Geometry: see drawing. Coordinates: mm, zero at the bounding-box minimum. A direction names the side the tool comes from. Give positions to 0.01 mm unless a question says otherwise; leave off trailing zeros. Write each loop counter-clockwise with the first axis right and the second up, starting at its lowest first coordinate (ties: lowest second). Pieces come first, ordered by that corner, then holes.
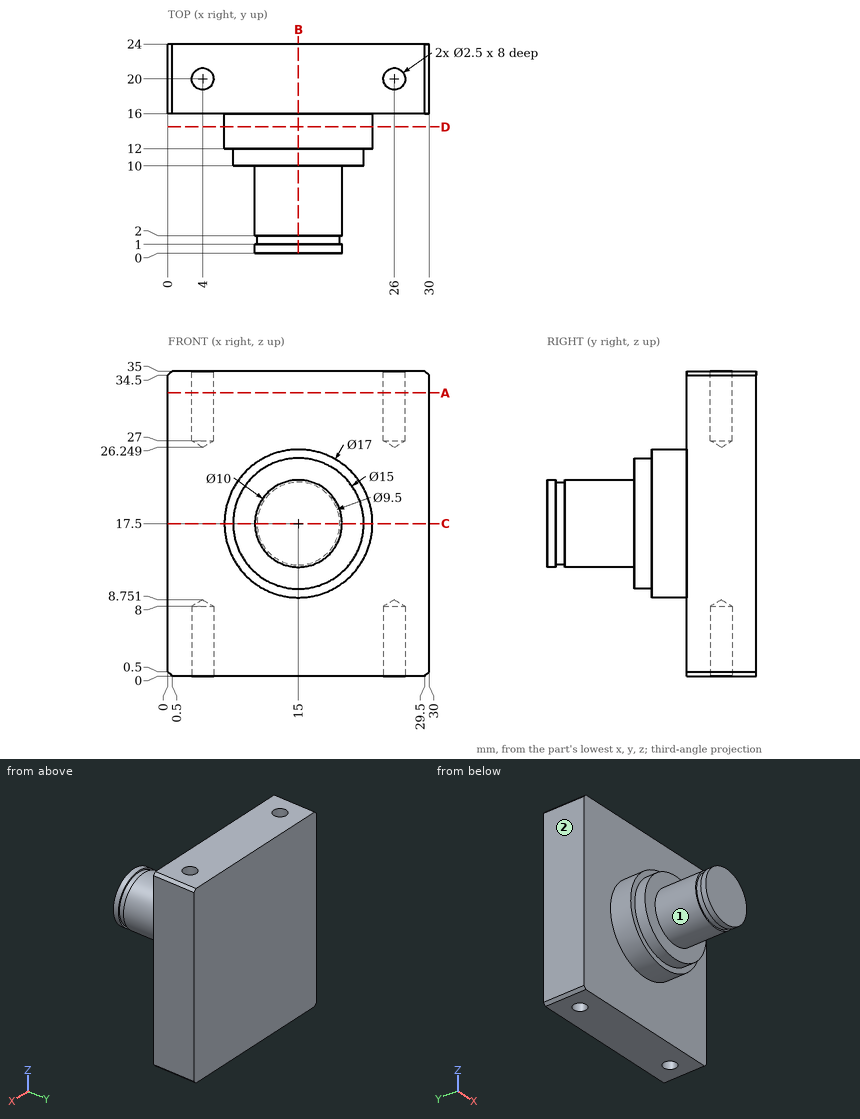
1. Section query B-B (x = 15). Return loops of the section in (y, z).
2. Line query: probe 1 along X at (y, z) = (20, 32.5); probe 2 along Y at (x, z) = (4, 32.25); probe 3 along Y at (x, z) = (6, 33). Output: solid intervals per line, ascending.
3. Access query for the marked faces 1 and 2. Directions: +Z, -Z, +X, -X, +Y, -Y. A direction counts if a zero-diameter tool reaches every point of the face in a straight line with its end or side. Return the directions, or none.
4. Section query D-D (y = 14.5). Return loops of the section in (x, z).
5. Pin query (flat end, axial travel): P1, Ø2, axis at x = 4, y = 20, coming from the +Z side; P2, Ø10, axis at x = 5.5, y = 5, coming from the +Z side; P3, Ø4, axis at y = 3.5, z = 15, coming from the +X side (3 decimals). Return the tip coordinate at first contact, or that it passes through.
6. Section query C-C (z = 17.5). Return loops of the section in (x, y), plus the area to 4 significant figures.
7. Section query A-A (z = 32.5). Return loops of the section in (x, y).
The answers:
1. outline: (0, 12.5) - (1, 12.5) - (1, 12.75) - (2, 12.75) - (2, 12.5) - (10, 12.5) - (10, 10) - (12, 10) - (12, 9) - (16, 9) - (16, 0) - (24, 0) - (24, 35) - (16, 35) - (16, 26) - (12, 26) - (12, 25) - (10, 25) - (10, 22.5) - (2, 22.5) - (2, 22.25) - (1, 22.25) - (1, 22.5) - (0, 22.5) - close
2. probe 1: x = 0 to 2.75, 5.25 to 24.75, 27.25 to 30
2. probe 2: y = 16 to 18.75, 21.25 to 24
2. probe 3: y = 16 to 24
3. face 1: -Y
3. face 2: +Z, -Z, -X, +Y, -Y
4. outline: circle Ø17 at (15, 17.5)
5. P1: stops at z = 26.85
5. P2: stops at z = 19.68
5. P3: stops at x = 19.975
6. outline: (0, 16) - (6.5, 16) - (6.5, 12) - (7.5, 12) - (7.5, 10) - (10, 10) - (10, 2) - (10.25, 2) - (10.25, 1) - (10, 1) - (10, 0) - (20, 0) - (20, 1) - (19.75, 1) - (19.75, 2) - (20, 2) - (20, 10) - (22.5, 10) - (22.5, 12) - (23.5, 12) - (23.5, 16) - (30, 16) - (30, 24) - (0, 24) - close
6. area: 437.5 mm2
7. outline: (0, 16) - (30, 16) - (30, 24) - (0, 24) - close; hole circle Ø2.5 at (4, 20); hole circle Ø2.5 at (26, 20)
